```python
from build123d import *

# Parameters (mm, degrees)
F0_R     = 2
F1_DEPTH = 2
F3_DEPTH = 15
F4_R     = 2


with BuildPart() as f1:
    # F0 (on Front) → F1 (new body)
    with BuildSketch(Plane.XZ):
        Polygon((40.190461, 17.494964), (-17.809539, 17.494964), (-17.809539, -11.005036), (-9.423875, -11.005036), (-9.423875, 12.596268), (31.804797, 12.596268), (31.804797, -11.005036), (40.190461, -11.005036), align=None)
        with Locations((-13.809539, -5.505036)):
            Circle(F0_R, mode=Mode.SUBTRACT)
        with Locations((36.190461, -5.505036)):
            Circle(F0_R, mode=Mode.SUBTRACT)
    extrude(amount=F1_DEPTH)

    # F2 (on face) → F3 (join)
    with BuildSketch(Plane.XZ):
        Polygon((31.804797, 7.494964), (40.190461, 7.494964), (40.190461, 17.494964), (-17.809539, 17.494964), (-17.809539, 7.494964), (-9.423875, 7.494964), (-9.423875, 12.596268), (31.804797, 12.596268), align=None)
    extrude(amount=-F3_DEPTH)

    # F4
    f4_edges = [f1.edges().sort_by_distance(p)[0] for p in [
        (-17.809539, 6.5, 17.494964),
        (40.190461, 6.5, 17.494964),
        (11.190461, -2, 12.596268),
        (31.804797, -2, 0.795616),
        (-9.423875, -2, 0.795616),
        (31.804797, 15, 10.045616),
        (11.190461, 15, 12.596268),
        (-9.423875, 15, 10.045616),
    ]]
    fillet(f4_edges, radius=F4_R)


solid = f1.part
```
Can you work these out from the model? Positions are in its coordinate system, mm. A direction names the side the tool comes from. Round coordinates to 2 decimals unless told otherwise and drop trailing zeros. Loops run counter-clockwise (first coordinate to the right, second up) from the corner with the lowest first, then second, coordinate; pieces in that order, holes last. Notation, with made-up numbers: (85.5, -29.5) -> (132.5, -29.5) arc R33 ccw to (132.5, 9.5) -> close; hole circle Ø8 at (85, 89.25). An arc over 180 degrees is marked (long way). One line per item, written item: value. Start each with the question number.
1. For faces 1 (the flat face through (31.805, 6, 10)), 2 (the cylindrical face through (-10.025, 14.43, 10.306)), 3 (the flat face through (-14, 7, 7.495)), 4 (the cylindrical face through (11.51, -1.4, 13.17)), which set-ups out of +Z, -Z, +X, -X, +Y, -Y let a thin tool reach every point of the face, with its end or its side?
2. If we section it at C-C, the plane x = 2: Write out the boundary of the cut face in (y, z), then the cut area to 3 significant figures.
3. If we section it at B-B, the plane y = 4: Write out the boundary of the cut face in (x, z), then the cut area to 3 significant figures.
4. For pin 1 (2.5 mm diameter, centred on x = -15.5, y = 9, fed in from -Z); pin 2 (9 mm diameter, centred on x = 37.5, z = -1.5, fed in from +Y); pin 3 (4.5 mm diameter, centred on x = -13.81, z = -5.51, fed in from -Y); pin 4 (5 mm diameter, centred on x = -0.5, y = 10.5, fed in from -Z), each with a flat end and sliding along its axis, tell me the tip position at first contact or that it passes through.
5. If we section it at D-D, the plane z = 9.25: Write out the boundary of the cut face in (x, y), then the cut area to 3 significant figures.
6. If I drill on probe 1 along X at (y, z) = (0.5, 8.5); probe 2 along Z at (x, y) = (-1.5, 10.25); probe 3 along Z at (x, y) = (-15, 9), over which ranges is the centre line in solid material (lowest first)?
7. If we section it at A-A, the plane z = -2: Write out the boundary of the cut face in (x, y), then the cut area to 3 significant figures.
Calculated:
1. face 1: -Z, +Y, -Y
1. face 2: -Z, +Y
1. face 3: -Z, +X, -X, +Y
1. face 4: -Z, -Y
2. outline: (-2, 14.6) arc R2 ccw to (0, 12.6) -> (13, 12.6) arc R2 ccw to (15, 14.6) -> (15, 17.49) -> (-2, 17.49) -> close
2. area: 81.6 mm²
3. outline: (-17.81, 7.49) -> (-9.42, 7.49) -> (-9.42, 12.6) -> (31.8, 12.6) -> (31.8, 7.49) -> (40.19, 7.49) -> (40.19, 15.49) arc R2 ccw to (38.19, 17.49) -> (-15.81, 17.49) arc R2 ccw to (-17.81, 15.49) -> close
3. area: 368 mm²
4. pin 1: stops at z = 7.49
4. pin 2: stops at y = 0
4. pin 3: stops at y = -2
4. pin 4: stops at z = 12.6
5. outline: (-17.81, -2) -> (-11.42, -2) arc R2 ccw to (-9.42, 0) -> (-9.42, 13) arc R2 ccw to (-11.42, 15) -> (-17.81, 15) -> close; (31.8, 0) arc R2 ccw to (33.8, -2) -> (40.19, -2) -> (40.19, 15) -> (33.8, 15) arc R2 ccw to (31.8, 13) -> close
5. area: 282 mm²
6. probe 1: x = -17.81 to -9.42, 31.8 to 40.19
6. probe 2: z = 12.6 to 17.49
6. probe 3: z = 7.49 to 17.49
7. outline: (-17.81, -2) -> (-11.42, -2) arc R2 ccw to (-9.42, 0) -> (-17.81, 0) -> close; (31.8, 0) arc R2 ccw to (33.8, -2) -> (40.19, -2) -> (40.19, 0) -> close
7. area: 31.8 mm²
